from build123d import *

# Parameters (mm, degrees)
SKETCH1_R             = 2
SKETCH1_R_2           = 0.9
BOSS_EXTRUDE1_DEPTH   = 3
BOSS_EXTRUDE1_2_DEPTH = 3
BOSS_EXTRUDE1_3_DEPTH = 3
SKETCH2_R             = 15
SKETCH2_R_2           = 1.95
BOSS_EXTRUDE2_DEPTH   = 4
SKETCH4_W             = 8
SKETCH4_H             = 3.3
CUT_EXTRUDE2_DEPTH    = 229.434345053
SKETCH5_R             = 6.75
CUT_EXTRUDE3_DEPTH    = 2.4
CUT_EXTRUDE5_DEPTH    = 1
SKETCH8_R             = 2.65
SKETCH8_R_2           = 1.95
BOSS_EXTRUDE3_DEPTH   = 21
SKETCH10_R            = 0.9
CUT_EXTRUDE6_DEPTH    = 230.514727196
SKETCH11_W            = 7
SKETCH11_H            = 2
CUT_EXTRUDE7_DEPTH    = 2


with BuildPart() as part:
    # Sketch1 → Boss-Extrude1 (new body)
    with BuildSketch(Plane.XY):
        with Locations((166.62, -116.13)):
            Circle(SKETCH1_R)
        with Locations((166.62, -116.13)):
            Circle(SKETCH1_R_2, mode=Mode.SUBTRACT)
    extrude(amount=BOSS_EXTRUDE1_DEPTH)



with BuildPart() as body_2:
    # Sketch1 → Boss-Extrude1 2 (new body)
    with BuildSketch(Plane.XY):
        with Locations((175.5, -100.75)):
            Circle(SKETCH1_R)
        with Locations((175.5, -100.75)):
            Circle(SKETCH1_R_2, mode=Mode.SUBTRACT)
    extrude(amount=BOSS_EXTRUDE1_2_DEPTH)


with BuildPart() as body_3:
    # Sketch1 → Boss-Extrude1 3 (new body)
    with BuildSketch(Plane.XY):
        with Locations((184.38, -116.13)):
            Circle(SKETCH1_R)
        with Locations((184.38, -116.13)):
            Circle(SKETCH1_R_2, mode=Mode.SUBTRACT)
    extrude(amount=BOSS_EXTRUDE1_3_DEPTH)


with BuildPart() as part_1:
    add(part.part)

    add(body_2.part)  # Boss-Extrude2 merges body 2

    add(body_3.part)  # Boss-Extrude2 merges body 3
    # Sketch2 → Boss-Extrude2 (add)
    with BuildSketch(Plane.XY.offset(3)):
        with Locations((175.5, -111)):
            Circle(SKETCH2_R)
        with Locations((175.5, -111)):
            Circle(SKETCH2_R_2, mode=Mode.SUBTRACT)
    extrude(amount=BOSS_EXTRUDE2_DEPTH)

    # Sketch4 → Cut-Extrude2 (cut, through all)
    with BuildSketch(Plane(origin=(0, 0, 3), x_dir=(-1, 0, 0), z_dir=(0, 0, -1))):
        with Locations((-175.5, -121.65)):
            Rectangle(SKETCH4_W, SKETCH4_H)
    extrude(amount=-CUT_EXTRUDE2_DEPTH, mode=Mode.SUBTRACT)

    # Sketch5 → Cut-Extrude3 (cut)
    with BuildSketch(Plane.XY.offset(7)):
        with Locations((175.5, -111)):
            Circle(SKETCH5_R)
    extrude(amount=-CUT_EXTRUDE3_DEPTH, mode=Mode.SUBTRACT)

    # Sketch6 → Cut-Extrude5 (cut)
    with BuildSketch(Plane(origin=(0, 0, 3), x_dir=(-1, 0, 0), z_dir=(0, 0, -1))):
        with BuildLine():
            Line((-173.55, -111), (-173.55, -120))
            ThreePointArc((-173.55, -120), (-175.5, -121.95), (-177.45, -120))
            Line((-177.45, -120), (-177.45, -111))
            ThreePointArc((-177.45, -111), (-175.5, -109.05), (-173.55, -111))
        make_face()
    extrude(amount=-CUT_EXTRUDE5_DEPTH, mode=Mode.SUBTRACT)

    # Sketch8 → Boss-Extrude3 (add)
    with BuildSketch(Plane.XY.offset(4.6)):
        with Locations(Location((175.5, -111, 0), (0, 0, 180))):
            Circle(SKETCH8_R)
        with Locations((175.5, -111)):
            Circle(SKETCH8_R_2, mode=Mode.SUBTRACT)
    extrude(amount=BOSS_EXTRUDE3_DEPTH)

    # Sketch10 → Cut-Extrude6 (cut, through all)
    with BuildSketch(Plane(origin=(0, 0, 3), x_dir=(-1, 0, 0), z_dir=(0, 0, -1))):
        with Locations(Location((-175.5, -100.75, 0), (0, 0, 180))):
            Circle(SKETCH10_R)
        with Locations(Location((-184.38, -116.13, 0), (0, 0, 180))):
            Circle(SKETCH10_R)
        with Locations(Location((-166.62, -116.13, 0), (0, 0, 180))):
            Circle(SKETCH10_R)
    extrude(amount=-CUT_EXTRUDE6_DEPTH, mode=Mode.SUBTRACT)

    # Sketch11 → Cut-Extrude7 (cut)
    with BuildSketch(Plane.XY.offset(25.6)):
        with Locations((175.5, -111)):
            Rectangle(SKETCH11_W, SKETCH11_H)
    extrude(amount=-CUT_EXTRUDE7_DEPTH, mode=Mode.SUBTRACT)


solid = part_1.part
Geometry: final body of the model. Coordinates: model frame, mm. A direction names the side the tool comes from. Give positions to 0.01 mm unless a question says otherwise; leave off trailing zeros. Write each loop counter-clockwise with the first axis right and the second up, starting at its lowest first coordinate (ties: lowest second). Pieces come first, ordered by that corner, then holes. Notation, with made-up numbers: M 64,67.25 L 111,67.25 A13 ccw 111,74.25 Z; hole C 74,21.5 d11. An arc over 180 degrees is marked long. Answer in a Markdown table with one row per item. Add a question column.
(1) Section C-C on y = -100.75. Return loops of the section in (x, z).
(2) Mould query, pull axis Y, two halves, no side actions, for faces 6 (the cylindrical face through (160.515, -110.34, 4.972)), 7 (the cylindrical face through (173.552, -110.914, 14.142)), 8 (the flat face through (176, -123.3, 5)), 9 (the flat face through (179, -111, 3)). Classes: +Y half, -Y half, draft (parallel to the pull), parting line (faces both ways), or undercut.
(3) Reachability of faces 1 (the flat face through (171.5, -122, 5)), 2 (the cylindrical face through (184.12, -114.147, 1.479)), 3 (the flat face through (173, -111, 23.6)), 4 (the cylindrical face through (178.61, -116.99, 5.82)), 5 (the flat face through (175.5, -113.2, 25.6)) from +Z, -Z, +X, -X, +Y, -Y: full face, straight path, thin tool, end or side. Return the list, or none.
(4) Section D-D on z = 12. Return loops of the section in (x, y).
(5) First-contact query: pin 1 (5 mm diameter, centred on x = 178, z = 16.5, fed in from +Y); pin 2 (5 mm diameter, centred on x = 165.5, y = -111.5, fed in from +Z); pin 3 (11 mm diameter, centred on x = 178, y = -111, fed in from +Z); pin 4 (1.7 mm diameter, centred on y = -121.5, z = 5.5, fed in from +X). Flat tips, straight axial feed; report the tip coordinate or a pass-through.
(6) Section A-A on x = 175.5. Return loops of the section in (y, z), and give its area (3 significant figures).
(7) Ray query, line 1 (Y direction, x = 175.5, z = 4.5); line 2 (Y direction, x = 175.5, z = 5.75); line 3 (Y direction, x = 175.5, z = 15.75). Return the intervals inside material, ascending.
(8) Section B-B on x = 166.62. Return loops of the section in (y, z), and give its area (3 significant figures).
Result set:
| question | item | result |
|---|---|---|
| 1 | outline | M 164.55,3 L 173.5,3 L 173.5,0 L 174.6,0 L 174.6,7 L 164.55,7 Z; M 176.4,0 L 177.5,0 L 177.5,3 L 186.45,3 L 186.45,7 L 176.4,7 Z |
| 2 | face 6 | parting line |
| 2 | face 7 | undercut |
| 2 | face 8 | undercut |
| 2 | face 9 | draft |
| 3 | face 1 | +Z, -Z |
| 3 | face 2 | -Z |
| 3 | face 3 | +Z, +X, -X |
| 3 | face 4 | +Z |
| 3 | face 5 | +Z, +X, -X, +Y, -Y |
| 4 | outline | C 175.5,-111 d5.3; hole C 175.5,-111 d3.9 |
| 5 | pin 1 | stops at y = -108.35 |
| 5 | pin 2 | stops at z = 7 |
| 5 | pin 3 | stops at z = 25.6 |
| 5 | pin 4 | stops at x = 186.98 |
| 6 | outline | M -126,3 L -123.3,3 L -123.3,7 L -126,7 Z; M -120,4 L -112.95,4 L -112.95,25.6 L -113.65,25.6 L -113.65,4.6 L -117.75,4.6 L -117.75,7 L -120,7 Z; M -109.05,3 L -102.75,3 L -102.75,0 L -101.65,0 L -101.65,7 L -104.25,7 L -104.25,4.6 L -108.35,4.6 L -108.35,25.6 L -109.05,25.6 Z; M -99.85,0 L -98.75,0 L -98.75,3 L -96,3 L -96,7 L -99.85,7 Z |
| 6 | area | 89.9 mm^2 |
| 7 | line 1 | y = -126 to -123.3, -120 to -112.95, -109.05 to -101.65, -99.85 to -96 |
| 7 | line 2 | y = -126 to -123.3, -120 to -117.75, -113.65 to -112.95, -109.05 to -108.35, -104.25 to -101.65, -99.85 to -96 |
| 7 | line 3 | y = -113.65 to -112.95, -109.05 to -108.35 |
| 8 | outline | M -123.09,3 L -118.13,3 L -118.13,0 L -117.03,0 L -117.03,7 L -123.09,7 Z; M -115.23,0 L -114.13,0 L -114.13,3 L -98.91,3 L -98.91,7 L -115.23,7 Z |
| 8 | area | 96.1 mm^2 |
